Design review of the part built by this model. Coordinates are the model's own, in mm. Coordinates: 2 decimals unless noted, no trailing zeros. Loops run counter-clockwise (first coordinate to the right, second up) from the corner with the lowest first, then second, coordinate; pieces in that order, holes last. Notation, with made-up numbers: M 61,49.25 L 117,49.25 A21 cw 117,59.25 Z; hole C 0,-16.75 d2. An arc over 180 degrees is marked long. Put each result on its own line as item: value. Start each with the question number.
(1) Take a section at B-B, the plane x = -21.19. Give the boundary of the cut face in (y, z).
(2) Take a section at C-C, the plane z = -22. Give the boundary of the cut face in (x, y), then the cut area to 3 significant figures.
(3) Clearance check with a flat-ended pin moving along its axis: pin 1 (1.7 mm diameter, centred on x = -14.19, z = -8, fed in from -Y). State where the tip first meets the part, or that it passes through.
(4) Take a section at A-A, the plane y = -0.6. Count the separate pieces of the cut face and the enclosed holes in it, then the cut area to 3 significant figures.
(5) For probe 1 along Z at (x, y) = (-7, -0.45); probe 2 along Z at (x, y) = (-21.19, -0.7); probe 3 along X at (y, z) = (-1, -24.25), list the stretches that pass through material, from the lowest coordinate up. Write a range as [from, to].
(6) Take a section at D-D, the plane x = -7.19. Give the boundary of the cut face in (y, z).
Autodesk Inventor part; units mm, degrees
ref_plane "YZ Plane" through (0, 0, 0) normal (1, 0, 0) x (0, 1, 0)
ref_plane "XZ Plane" through (0, 0, 0) normal (0, 1, 0) x (-1, 0, 0)
ref_plane "XY Plane" through (0, 0, 0) normal (0, 0, 1) x (1, 0, 0)
sketch "Sketch1" plane through (0, 0, 0) normal (0, 1, 0) x (-1, 0, 0)
  line L0 (-0.4496, -30) -> (-0.4496, 0)
  line L1 (-54.9089, 0) -> (-54.9089, -30)
  circle A0 centre (-20.1543, -27.5) radius 1.05
  circle A1 centre (-20.1543, -7.5) radius 1.05
  circle A2 centre (-35.2043, -27.5) radius 1.05
  circle A3 centre (-35.2043, -7.5) radius 1.05
  circle A4 centre (-69.5486, -15) radius 2.6
  circle A5 centre (14.19, -15) radius 3.6
  circle A6 centre (7.19, -15) radius 1.05
  circle A7 centre (14.19, -22) radius 1.05
  circle A8 centre (21.19, -15) radius 1.05
  circle A9 centre (14.19, -8) radius 1.05
  circle A10 centre (-69.5486, -22) radius 1.05
  circle A11 centre (-62.5486, -15) radius 1.05
  circle A12 centre (-69.5486, -8) radius 1.05
  circle A13 centre (-76.5486, -15) radius 1.05
  line L2 (-72.585, -24.4859) -> (-55.3586, -30)
  line L3 (0, -30) -> (17.2264, -24.4859)
  arc A14 (-72.585, -5.5141) -> (-72.585, -24.4859) centre (-69.5486, -15) ccw
  arc A15 (17.2264, -24.4859) -> (17.2264, -5.5141) centre (14.19, -15) ccw
  line L4 (-55.3586, 0) -> (-72.585, -5.5141)
  line L5 (17.2264, -5.5141) -> (0, 0)
  line L6 (-55.3586, 0) -> (0, 0)
  line L7 (0, -30) -> (-55.3586, -30)
  line L8 (-55.3586, -30) -> (-55.3586, 0)
  line L9 (-54.4593, 0) -> (-54.4593, -30)
  line L10 (-0.8993, -30) -> (-0.8993, 0)
  line L11 (0, 0) -> (0, -30)
extrude "Extrusion1" add sketch "Sketch1" against normal blind 1.5
sketch "Sketch2" plane through (0, 0, 0) normal (0, 1, 0) x (1, 0, 0)
  line L0 (0, 0) -> (0, 30)
  line L1 (0.4496, 30) -> (0.4496, 0)
  line L2 (0.8993, 30) -> (0.8993, 0)
  line L3 (54.4593, 0) -> (54.4593, 30)
  line L4 (54.9089, 0) -> (54.9089, 30)
  line L5 (55.3586, 30) -> (55.3586, 0)
properties part number "axis_14_bottom_frame"
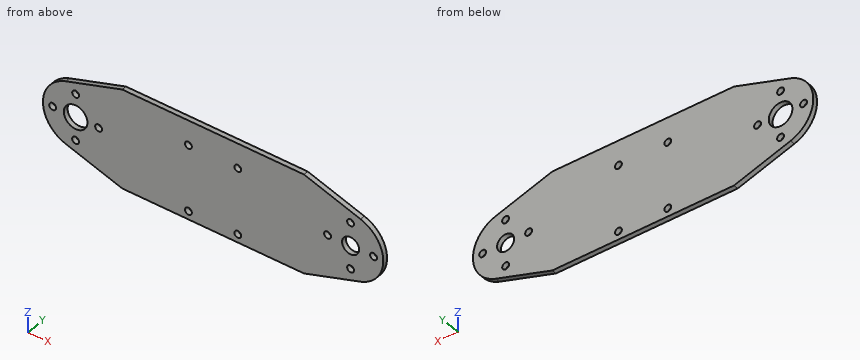
Computed values:
1. outline: M -1.5,-22.09 L 0,-22.09 L 0,-16.05 L -1.5,-16.05 Z; M -1.5,-13.95 L 0,-13.95 L 0,-7.91 L -1.5,-7.91 Z
2. outline: M -21.28,-1.5 L -15.24,-1.5 L -15.24,0 L -21.28,0 Z; M -13.14,-1.5 L 68.5,-1.5 L 68.5,0 L -13.14,0 Z; M 70.6,-1.5 L 76.63,-1.5 L 76.63,0 L 70.6,0 Z
2. area: 141 mm^2
3. pin 1: passes through
4. separate pieces: 1
4. enclosed holes: 14
4. area: 2,590 mm^2
5. probe 1: z = [-27.76, -16.03], [-13.97, -2.24]
5. probe 2: z = [-22.09, -16.05], [-13.95, -7.91]
5. probe 3: x = [-17.88, 73.24]
6. outline: M -1.5,-27.7 L 0,-27.7 L 0,-16.05 L -1.5,-16.05 Z; M -1.5,-13.95 L 0,-13.95 L 0,-2.3 L -1.5,-2.3 Z
